The listing builds one solid part. Answer for the finished solid, in the listing's coordinates (mm). A direction names the side the tool comes from. Round coordinates to 2 decimals unless told otherwise and drop trailing zeros. Write each loop counter-clockwise with the first axis right and the second up, starting at its lowest first coordinate (ties: lowest second). Pieces come first, ordered by that corner, then holes. Notation, with made-up numbers: (-11.75, 4) - (23.25, 4) arc R17 ccw to (23.25, 29) - close; hole circle Ø2 at (69.25, 10). An arc over 180 degrees is marked (long way). Use a Markdown table: item, result. Add a question column.
1) A cutting plane is placed at B-B (z = 0.5). Give the vertices of the cut face in (x, y).
2) A tool of negligible diameter and unlimited length cuts with its end or side. For faces 1 (the flat face through (-0.1, -5.5, -1.4)), 2 (the flat face through (-0.01, 0, 1.4)), 3 (the cylindrical face through (-0.27, 6.66, -1.22)), 4 (the flat face through (-0.1, 0, -1.4)), 5 (the flat face through (-0.01, -5.5, 1.4)), from which of +Z, -Z, +X, -X, +Y, -Y can it reach the whole face along a straight path? Write none if from no direction.
3) A cutting plane is placed at A-A (x = 0). Give the vertices of the cut face in (y, z), then the cut area to 3 significant figures.
4) Determine the mould class of faces 6 (the cylindrical face through (0.02, -2.71, 1.75)), 7 (the flat face through (-1.25, -3, 0)), 8 (the cylindrical face through (-0.02, -2.71, -1.75)), 9 (the cylindrical face through (-0.27, -9.56, -1.22)) for opening direction Z: +Z half, -Z half, draft (parallel to the pull), parting line (faces both ways), or undercut.
5) Find the intervals of material crossed by probe 1 along Y at (x, z) = (-0.5, 1.5); probe 2 along X at (y, z) = (-8.25, 0.05); probe 3 along Z at (x, y) = (-0.65, 4.25), in increasing order. Write a range as from..to.
6) A cutting plane is placed at C-C (y = -7). Give the vertices of the cut face in (x, z).
```python
from build123d import *

# Parameters (mm, degrees)
F1_DEPTH = 5.5
F2_R     = 1.25
F3_DEPTH = 13.5


with BuildPart() as f1:
    # F0 (on Front) → F1 (new body)
    with BuildSketch(Plane.XZ):
        with BuildLine():
            Line((-1.25, 1.224745), (-1.25, -1.224745))
            ThreePointArc((-1.25, -1.224745), (0, -1.75), (1.25, -1.224745))
            Line((1.25, -1.224745), (1.25, 1.224745))
            ThreePointArc((1.25, 1.224745), (0, 1.75), (-1.25, 1.224745))
        make_face()
    extrude(amount=F1_DEPTH)

    # F2 (on Front) → F3 (join, symmetric)
    with BuildSketch(Plane.XZ):
        Circle(F2_R)
    extrude(amount=F3_DEPTH, both=True)


solid = f1.part
```
Entries:
| question | item | result |
|---|---|---|
| 1 | outline | (-1.25, -5.5) - (-1.15, -5.5) - (-1.15, -13.5) - (1.15, -13.5) - (1.15, -5.5) - (1.25, -5.5) - (1.25, 0) - (1.15, 0) - (1.15, 13.5) - (-1.15, 13.5) - (-1.15, 0) - (-1.25, 0) - close |
| 2 | face 1 | -Z, -Y |
| 2 | face 2 | +Z, +Y |
| 2 | face 3 | +Y |
| 2 | face 4 | -Z, +Y |
| 2 | face 5 | +Z, -Y |
| 3 | outline | (-13.5, -1.25) - (-5.5, -1.25) - (-5.5, -1.75) - (0, -1.75) - (0, -1.25) - (13.5, -1.25) - (13.5, 1.25) - (0, 1.25) - (0, 1.75) - (-5.5, 1.75) - (-5.5, 1.25) - (-13.5, 1.25) - close |
| 3 | area | 73.0 mm² |
| 4 | face 6 | +Z half |
| 4 | face 7 | draft |
| 4 | face 8 | -Z half |
| 4 | face 9 | parting line |
| 5 | probe 1 | y = -5.5..0 |
| 5 | probe 2 | x = -1.25..1.25 |
| 5 | probe 3 | z = -1.07..1.07 |
| 6 | outline | circle Ø2.5 at (0, 0) |
